from build123d import *

# Parameters (mm, degrees)
ESQUISSE1_R             = 12
BOSS_EXTRU_1_DEPTH      = 2
BOSS_EXTRU_2_DEPTH      = 30
BOSS_EXTRU_3_DEPTH      = 0.45
ENL_V_MAT_EXTRU_1_REACH = 71


with BuildPart() as part:
    # Esquisse1 → Boss.-Extru.1 (new body)
    with BuildSketch(Plane.XY):
        Circle(ESQUISSE1_R)
        with BuildLine():
            ThreePointArc((-8.473394023, 3.033412884), (-8.624994546, 2.570888774), (-8.751368421, 2.10084525))
            ThreePointArc((-8.751368421, 2.10084525), (-8.012421402, 0.895043731), (-6.806619883, 1.63399075))
            ThreePointArc((-6.806619883, 1.63399075), (-6.708329091, 1.999580157), (-6.590417574, 2.359321132))
            ThreePointArc((-6.590417574, 2.359321132), (-7.194859923, 3.637855233), (-8.473394023, 3.033412884))
        make_face(mode=Mode.SUBTRACT)
        with BuildLine():
            ThreePointArc((3.033412884, 8.473394023), (2.570888774, 8.624994546), (2.10084525, 8.751368421))
            ThreePointArc((2.10084525, 8.751368421), (0.895043731, 8.012421402), (1.63399075, 6.806619883))
            ThreePointArc((1.63399075, 6.806619883), (1.999580157, 6.708329091), (2.359321132, 6.590417574))
            ThreePointArc((2.359321132, 6.590417574), (3.637855233, 7.194859923), (3.033412884, 8.473394023))
        make_face(mode=Mode.SUBTRACT)
        with BuildLine():
            ThreePointArc((8.473394023, -3.033412884), (8.624994546, -2.570888774), (8.751368421, -2.10084525))
            ThreePointArc((8.751368421, -2.10084525), (8.012421402, -0.895043731), (6.806619883, -1.63399075))
            ThreePointArc((6.806619883, -1.63399075), (6.708329091, -1.999580157), (6.590417574, -2.359321132))
            ThreePointArc((6.590417574, -2.359321132), (7.194859923, -3.637855233), (8.473394023, -3.033412884))
        make_face(mode=Mode.SUBTRACT)
        with BuildLine():
            ThreePointArc((-3.033412884, -8.473394023), (-2.570888774, -8.624994546), (-2.10084525, -8.751368421))
            ThreePointArc((-2.10084525, -8.751368421), (-0.895043731, -8.012421402), (-1.63399075, -6.806619883))
            ThreePointArc((-1.63399075, -6.806619883), (-1.999580157, -6.708329091), (-2.359321132, -6.590417574))
            ThreePointArc((-2.359321132, -6.590417574), (-3.637855233, -7.194859923), (-3.033412884, -8.473394023))
        make_face(mode=Mode.SUBTRACT)
    extrude(amount=BOSS_EXTRU_1_DEPTH)

    # Esquisse2 → Boss.-Extru.2 (add)
    with BuildSketch(Plane.XY.offset(2)):
        with BuildLine():
            Line((-2, 4), (2, 4))
            ThreePointArc((2, 4), (3.414213562, 3.414213562), (4, 2))
            Line((4, 2), (4, -2))
            ThreePointArc((4, -2), (3.414213562, -3.414213562), (2, -4))
            Line((2, -4), (-2, -4))
            ThreePointArc((-2, -4), (-3.414213562, -3.414213562), (-4, -2))
            Line((-4, -2), (-4, 2))
            ThreePointArc((-4, 2), (-3.414213562, 3.414213562), (-2, 4))
        make_face()
    extrude(amount=BOSS_EXTRU_2_DEPTH)


with BuildPart() as body_2:
    # Esquisse3 → Boss.-Extru.3 (new, symmetric)
    with BuildSketch(Plane(origin=(0, 0, 0), x_dir=(0, 0, -1), z_dir=(1, 0, 0))):
        with BuildLine():
            Line((-11.963767642, -29), (-22.036232358, -29))
            Line((-22.036232358, -29), (-18.266617818, -58.387853285))
            ThreePointArc((-18.266617818, -58.387853285), (-17.638228926, -58.70410685), (-17, -59))
            ThreePointArc((-17, -59), (-16.361771074, -58.70410685), (-15.733382182, -58.387853285))
            Line((-15.733382182, -58.387853285), (-11.963767642, -29))
        make_face()
    extrude(amount=BOSS_EXTRU_3_DEPTH, both=True)


    add(part.part)  # lissage1 joins it to this body
    # loft from a face of the part (lissage1)
    loft([body_2.faces().sort_by_distance((0, -29, 17))[0], body_2.faces().sort_by_distance((0, -4, 17))[0]])

    # Enlèv. mat.-Extru.1: up to this plane
    enl_v_mat_extru_1_end = Plane(origin=(-2.239391778, -0.13884229, 0), z_dir=(-0.998083523435423, -0.061881178452996184, 0))
    # Esquisse5 → Enlèv. mat.-Extru.1 (cut, up to the surface)
    with BuildSketch(Plane.ZY.offset(-4), mode=Mode.PRIVATE) as enl_v_mat_extru_1_sk1:
        with BuildLine():
            ThreePointArc((32, -4), (24.618937512, -15.543805649), (22.036232358, -29))
            Line((22.036232358, -29), (32, -4))
        make_face()
    enl_v_mat_extru_1_tool1 = split(extrude(enl_v_mat_extru_1_sk1.sketch, amount=ENL_V_MAT_EXTRU_1_REACH, mode=Mode.PRIVATE), bisect_by=enl_v_mat_extru_1_end, keep=Keep.BOTH, mode=Mode.PRIVATE)
    add(enl_v_mat_extru_1_tool1.solids().sort_by_distance((4, -16.116333, 26.055461))[0], mode=Mode.SUBTRACT)
    # Esquisse5 → Enlèv. mat.-Extru.1 (cut, up to the surface)
    with BuildSketch(Plane.ZY.offset(-4), mode=Mode.PRIVATE) as enl_v_mat_extru_1_sk2:
        with BuildLine():
            Line((32, -4), (22.036232358, -29))
            ThreePointArc((22.036232358, -29), (58.381754034, -65.345521676), (94.727275711, -29))
            ThreePointArc((94.727275711, -29), (71.837948385, 4.762816522), (32, -4))
        make_face()
    enl_v_mat_extru_1_tool2 = split(extrude(enl_v_mat_extru_1_sk2.sketch, amount=ENL_V_MAT_EXTRU_1_REACH, mode=Mode.PRIVATE), bisect_by=enl_v_mat_extru_1_end, keep=Keep.BOTH, mode=Mode.PRIVATE)
    add(enl_v_mat_extru_1_tool2.solids().sort_by_distance((4, -29.146557, 58.74948))[0], mode=Mode.SUBTRACT)
    # Esquisse5 → Enlèv. mat.-Extru.1 (cut, up to the surface)
    with BuildSketch(Plane.ZY.offset(-4), mode=Mode.PRIVATE) as enl_v_mat_extru_1_sk3:
        with BuildLine():
            Line((2, -4), (11.963767642, -29))
            ThreePointArc((11.963767642, -29), (9.381062488, -15.543805649), (2, -4))
        make_face()
    enl_v_mat_extru_1_tool3 = split(extrude(enl_v_mat_extru_1_sk3.sketch, amount=ENL_V_MAT_EXTRU_1_REACH, mode=Mode.PRIVATE), bisect_by=enl_v_mat_extru_1_end, keep=Keep.BOTH, mode=Mode.PRIVATE)
    add(enl_v_mat_extru_1_tool3.solids().sort_by_distance((4, -16.116333, 7.944539))[0], mode=Mode.SUBTRACT)


solid = body_2.part
Work out the finished part from the listing and answer in its coordinate system (mm). A direction names the side the tool comes from. Give positions to 0.01 mm unless a question says otherwise; leave off trailing zeros. Loops run counter-clockwise (first coordinate to the right, second up) from the corner with the lowest first, then second, coordinate; pieces in that order, holes last. Notation, with made-up numbers: (80.25, 88) -> (112.25, 88) arc R15 cw to (112.25, 93) -> close; hole circle Ø6 at (37, 76.25). An arc over 180 degrees is marked (long way). Use a Markdown table: item, result. Add a question column.
1. For faces 1 (the flat face through (-4, 0, 17)), 2 (the flat face through (-0.45, -40, 17)), 3 (the cylindrical face through (-3.4, -3.43, 16.79)), 4 (the flat face through (4, 0, 17)), determine the directions among +Z, -Z, +X, -X, +Y, -Y from which every point of the face is accessible in a straight line to the end or side of a thin tool.
2. Determine the mould class of faces 5 (the cylindrical face through (-7.17, 3.63, 0.99)), 6 (the flat face through (0, 0, 32)), 7 (the cylindrical face through (0.9, 8.03, 0.99)), 8 (the cylindrical face through (-3.43, 3.4, 16.79)) for opening direction Y: released by +Y, released by -Y, zero draft, split by the parting line, or undercut.
3. Section C-C on y = -39.5 is taken. Determine the outline of the cut face in (x, z).
4. Section A-A on x = -7.75 is taken. Determine the outline of the cut face in (y, z), and give its area (3 significant figures).
5. Section D-D on y = -53.5 is taken. Determine the outline of the cut face in (x, z), and give its area (3 significant figures).
6. Find the intervals of material crossed by probe 1 along X at (y, z) = (-10, 24); probe 2 along Z at (x, y) = (-4.25, -3); probe 3 along X at (y, z) = (-35, 13.5), in increasing order.
7. Flat-ended cylindrical pins translate along their axes: pin 1 Ø5 at (x, y) = (0.5, -49) entering from +Z; pin 2 Ø4 at (x, y) = (0, -32.5) entering from +Z; pin 3 Ø5 at (x, y) = (0.5, -51.5) entering from -Z. Find the tip coordinate at first contact, or state that the pin passes through.
8. Section B-B on y = 0 is taken. Determine the outline of the cut face in (x, z).
Results below:
| question | item | result |
|---|---|---|
| 1 | face 1 | +Z, -X, +Y, -Y |
| 1 | face 2 | +Z, -Z, -X, -Y |
| 1 | face 3 | +Z, -X, -Y |
| 1 | face 4 | +Z, +X, +Y, -Y |
| 2 | face 5 | undercut |
| 2 | face 6 | zero draft |
| 2 | face 7 | undercut |
| 2 | face 8 | released by +Y |
| 3 | outline | (-0.45, 13.31) -> (0.45, 13.31) -> (0.45, 20.69) -> (-0.45, 20.69) -> close |
| 4 | outline | (-9.16, 0) -> (0.87, 0) -> (0.87, 2) -> (-9.16, 2) -> close; (3.67, 0) -> (9.16, 0) -> (9.16, 2) -> (3.67, 2) -> close |
| 4 | area | 31.0 mm^2 |
| 5 | outline | (-0.45, 15.11) -> (0.45, 15.11) -> (0.45, 18.89) -> (-0.45, 18.89) -> close |
| 5 | area | 3.41 mm^2 |
| 6 | probe 1 | x = -1.63 to 1.63 |
| 6 | probe 2 | z = 0 to 2 |
| 6 | probe 3 | x = -0.45 to 0.45 |
| 7 | pin 1 | stops at z = 19.79 |
| 7 | pin 2 | stops at z = 21.84 |
| 7 | pin 3 | stops at z = 14.53 |
| 8 | outline | (-12, 0) -> (12, 0) -> (12, 2) -> (4, 2) -> (4, 32) -> (-4, 32) -> (-4, 2) -> (-12, 2) -> close |
